Geometry check sheet. Reference: the model listing, model coordinates, mm. A direction names the side the tool comes from. Round coordinates to 2 decimals unless told otherwise and drop trailing zeros. Loops run counter-clockwise (first coordinate to the right, second up) from the corner with the lowest first, then second, coordinate; pieces in that order, holes last. Notation, with made-up numbers: M 38,87.5 L 74,87.5 A18 ccw 74,114.5 Z; hole C 83,50.25 d9. An arc over 180 degrees is marked long. Answer in a Markdown table with one row per item. Add a question column.
```python
from build123d import *

# Parameters (mm, degrees)
SKETCH_1_W          = 60
SKETCH_1_H          = 21
EXTRUDE_1_DEPTH     = 2
SKETCH_2_W          = 2
SKETCH_2_H          = 7
CUT_EXTRUDE_1_DEPTH = 64.600314465
SKETCH_3_W          = 7
SKETCH_3_H          = 2
CUT_EXTRUDE_2_DEPTH = 64.600314465
SKETCH_5_R          = 0.5
CUT_EXTRUDE_3_DEPTH = 64.600314465


with BuildPart() as part:
    # 草图1 → 凸台-拉伸1 (new body)
    with BuildSketch(Plane.XY):
        with Locations((30, 10.5)):
            Rectangle(SKETCH_1_W, SKETCH_1_H)
    extrude(amount=EXTRUDE_1_DEPTH)

    # 草图2 → 切除-拉伸1 (cut, through all)
    with BuildSketch(Plane.XY.offset(2)):
        with Locations((1, 10.5)):
            Rectangle(SKETCH_2_W, SKETCH_2_H)
        with Locations((59, 10.5)):
            Rectangle(SKETCH_2_W, SKETCH_2_H)
    extrude(amount=-CUT_EXTRUDE_1_DEPTH, mode=Mode.SUBTRACT)

    # 草图3 → 切除-拉伸2 (cut, through all)
    with BuildSketch(Plane.XY.offset(2)):
        with Locations((13.5, 20)):
            Rectangle(SKETCH_3_W, SKETCH_3_H)
        with Locations((30, 20)):
            Rectangle(SKETCH_3_W, SKETCH_3_H)
        with Locations((46.5, 20)):
            Rectangle(SKETCH_3_W, SKETCH_3_H)
    extrude(amount=-CUT_EXTRUDE_2_DEPTH, mode=Mode.SUBTRACT)

    # 草图5 → 切除-拉伸3 (cut, through all)
    with BuildSketch(Plane.XY.offset(2)):
        with Locations((2, 7)):
            Circle(SKETCH_5_R)
    cut_extrude_3 = extrude(amount=-CUT_EXTRUDE_3_DEPTH, mode=Mode.SUBTRACT)

    # 草图阵列1: 切除-拉伸3 at 9 more places
    with Locations((0, 7, 0), (8, 12, 0), (15, 12, 0), (24.5, 12, 0), (31.5, 12, 0), (41, 12, 0), (48, 12, 0), (56, 7, 0), (56, 0, 0)):
        add(cut_extrude_3, mode=Mode.SUBTRACT)


solid = part.part
```
1) Thickness scan on L1, parallel to Y at x = 13, z = 0.95; L2, parallel to X at y = 12.75, z = 0.2. Record the ranges inside material, lowest first. Write a range as [from, to].
2) Set-up check for faces 4 (the flat face through (58, 10, 1)), 5 (the flat face through (1, 14, 1)), 6 (the flat face through (10, 20, 1)): record each of +Z, -Z, +X, -X, +Y, -Y from which the full face is reachable in a straight line by a thin tool's end or side.
3) Draft check along X on faces 1 (the cylindrical face through (17.3, 18.6, 1)), 2 (the flat face through (30, 0, 1)), 3 (the flat face through (60, 3, 1)). Enter one of: +X half, -X half, draft (parallel to the pull), parting line (faces both ways), or undercut.
4) Cross-section at B-B, the plane x = 14.5. Record the boundary of the cut face in (y, z).
5) Go/stop test with flat-tipped pins: pin 1 (1 mm diameter, centred on x = 29, z = 1, fed in from +Y); pin 2 (6 mm diameter, centred on x = 36, y = 3, fed in from -Z); pin 3 (1 mm diameter, centred on y = 10, z = 0.5, fed in from -X). Record where each tip stops, or that it passes through.
Worked answers:
| question | item | result |
|---|---|---|
| 1 | L1 | y = [0, 19] |
| 1 | L2 | x = [2, 58] |
| 2 | face 4 | +Z, -Z, +X |
| 2 | face 5 | +Z, -Z, -X |
| 2 | face 6 | +Z, -Z, +Y |
| 3 | face 1 | undercut |
| 3 | face 2 | draft |
| 3 | face 3 | +X half |
| 4 | outline | M 0,0 L 19,0 L 19,2 L 0,2 Z |
| 5 | pin 1 | stops at y = 19 |
| 5 | pin 2 | stops at z = 0 |
| 5 | pin 3 | stops at x = 2 |
